Autodesk Inventor part; units mm, degrees
ref_plane "YZ Plane" through (0, 0, 0) normal (1, 0, 0) x (0, 1, 0)
ref_plane "XZ Plane" through (0, 0, 0) normal (0, 1, 0) x (-1, 0, 0)
ref_plane "XY Plane" through (0, 0, 0) normal (0, 0, 1) x (1, 0, 0)
sketch "Sketch1" plane through (0, 0, 0) normal (0, 0, 1) x (1, 0, 0)
  circle A0 centre (0, 0) radius 5.0165
  dimension "d0" = 10.033
extrude "Extrusion1" add sketch "Sketch1" against normal blind 1.27
sketch "Sketch2" plane through (0, 0, -1.27) normal (0, 0, -1) x (-1, 0, 0)
  circle A0 centre (0, 0) radius 5.0165
  line L0 (-3.1496, -3.1496) -> (3.1496, -3.1496)
  line L1 (3.1496, -3.1496) -> (3.1496, 3.1496)
  line L2 (3.1496, 3.1496) -> (-3.1496, 3.1496)
  line L3 (-3.1496, 3.1496) -> (-3.1496, -3.1496)
  point P0 (0, 3.1496)
  point P1 (-3.1496, 0)
  dimension "d3" = 6.2992
extrude "Extrusion2" add sketch "Sketch2" along normal blind 3.81 contours L3 L2 L1 L0
fillet "Fillet1" radius 0.508 8 edges at (3.1496, 3.1496, -3.175) (-3.1496, 3.1496, -3.175) (-3.1496, -3.1496, -3.175) (3.1496, -3.1496, -3.175) (3.1496, 0, -5.08) (0, 3.1496, -5.08) (-3.1496, 0, -5.08) (0, -3.1496, -5.08)
sketch "Sketch3" plane through (0, 0, 0) normal (0, 0, 1) x (1, 0, 0)
  circle A0 centre (0, 0) radius 5.0165
hole "Hole1" at (0, 0, 0) direction (0, 0, -1) diameter 4.064 end through all
properties part number "Free Spinning Gear Insert" material "Acetal Resin, White"
CAD build for the part. Positions are in the model's coordinates, mm. A direction names the side the tool comes from. Coordinates: 2 decimals unless noted, no trailing zeros. Write each loop counter-clockwise with the first axis right and the second up, starting at its lowest first coordinate (ties: lowest second). Pieces come first, ordered by that corner, then holes. Notation, with made-up numbers: (30.5, -27.5) -> (80.5, -27.5) arc R31 ccw to (80.5, 10.5) -> close; hole circle Ø8 at (76, 5.25). An arc over 180 degrees is marked (long way). Return JSON: item names as keys, results as strings. Group by question number.
Q1. Drill centre lines: line 1 (X direction, y = 0, z = -1.85); line 2 (Y direction, x = 0, z = -1). Where is each one in solid material? Low to high.
Q2. Cut at D-D, the plane y = 2.25. Give the cut face in (x, z).
Q3. Which spindle directions (+Z, -Z, +X, -X, +Y, -Y) get a long thin tool onto all of the face, cutting with end or side? Do faces 1 (the face through (0, -3.15, -3)), 2 (the face through (-3.15, 0, -3)), 3 (the face through (-0.1, -3.3, -1.27)). Say none if no direction does.
Q4. Cut at C-C, the plane z = -2.85. Give the cut face in (x, y).
Q5. Cut at A-A, the plane x = 0. Give the cut face in (y, z), then the cut area to 3 significant figures.
Q6. Pull direction Y, two halves, no side cores. Call faces 4 (the face through (0, 3.15, -3)), 5 (the face through (3.15, 0, -3)), 6 (the face through (-1.087, -4.897, -0.626)), 7 (the face through (1.984, 0.44, -2.576)): released by +Y, released by -Y, zero draft, split by the parting line, or undercut.
Q7. Flat gauge pins, fed straight in: pin 1 (1.7 mm diameter, centred on x = -1, z = -3.5, fed in from +Y); pin 2 (2.5 mm diameter, centred on y = 1, z = -3.5, fed in from +X); pin 3 (1.5 mm diameter, centred on x = -3.5, z = -3, fed in from -Y). Where does each tip first touch, or does it go through?
Returned:
{
 "1": {"line 1": "x = -3.15 to -2.03, 2.03 to 3.15", "line 2": "y = -5.02 to -2.03, 2.03 to 5.02"},
 "2": {"outline": "(-4.48, -1.27) -> (-3.15, -1.27) -> (-3.15, -4.57) arc R0.51 ccw to (-2.64, -5.08) -> (2.64, -5.08) arc R0.51 ccw to (3.15, -4.57) -> (3.15, -1.27) -> (4.48, -1.27) -> (4.48, 0) -> (-4.48, 0) -> close"},
 "3": {"face 1": "-Z, +X, -X, -Y", "face 2": "-Z, -X, +Y, -Y", "face 3": "-Z"},
 "4": {"outline": "(-3.15, -2.64) arc R0.51 ccw to (-2.64, -3.15) -> (2.64, -3.15) arc R0.51 ccw to (3.15, -2.64) -> (3.15, 2.64) arc R0.51 ccw to (2.64, 3.15) -> (-2.64, 3.15) arc R0.51 ccw to (-3.15, 2.64) -> close; hole circle Ø4.06 at (0, 0)"},
 "5": {"outline": "(-5.02, -1.27) -> (-3.15, -1.27) -> (-3.15, -4.57) arc R0.51 ccw to (-2.64, -5.08) -> (-2.03, -5.08) -> (-2.03, 0) -> (-5.02, 0) -> close; (2.03, -5.08) -> (2.64, -5.08) arc R0.51 ccw to (3.15, -4.57) -> (3.15, -1.27) -> (5.02, -1.27) -> (5.02, 0) -> (2.03, 0) -> close", "area": "16.0 mm2"},
 "6": {"face 4": "released by +Y", "face 5": "zero draft", "face 6": "split by the parting line", "face 7": "undercut"},
 "7": {"pin 1": "stops at y = 3.15", "pin 2": "stops at x = 3.15", "pin 3": "stops at y = -3.14"}
}
